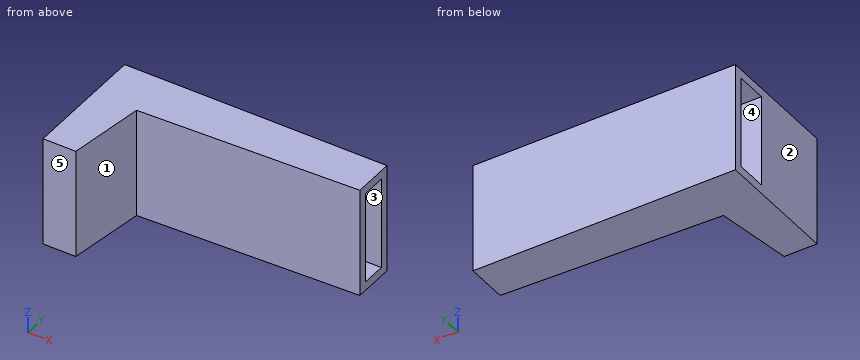
from build123d import *

# Parameters (mm, degrees)
PAD001_DEPTH = 8.4
PAD_DEPTH    = 10


with BuildPart() as pegcutoutpad:
    # Sketch001 → Pad001 (new body)
    with BuildSketch(Plane.XY.offset(0.8)):
        Polygon((20, -0.8), (-4, -0.8), (-4, -3.67), (0, -3.67), (20, -3.016154), align=None)
    extrude(amount=PAD001_DEPTH)


with BuildPart() as pegcut:
    # Sketch → Pad (new body)
    with BuildSketch(Plane.XY):
        Polygon((20, 0), (20, -3.816154), (0, -4.47), (-1, -11.47), (-4, -11.47), (-4, 0), align=None)
    extrude(amount=PAD_DEPTH)

    # Cut: cut PegCutOutPad
    add(pegcutoutpad.part, mode=Mode.SUBTRACT)


solid = pegcut.part
Part model, mm, in its own coordinate system. Face numbers are marked on the shaded views. A direction names the side the tool comes from. Give positions to 0.01 mm unless a question says otherwise; leave off trailing zeros. Order: outer loops, then holes, each group sorted by start corner. A loop starts at its lowest first (then second) coordinate and runs counter-clockwise, first axis right, second up. Notation, with made-up numbers: (-23, 41) -> (-8, 41) arc R16 cw to (-8, 50) -> close; hole circle Ø8 at (-40, 21). An arc over 180 degrees is marked (long way). Use one line per item in the form item = value.
(1) Pull direction Y, two halves, no side cores. Call the marked faces 1, 2 and 3: +Y half, -Y half, draft (parallel to the pull), parting line (faces both ways), or undercut.
Solution:
face_1 = -Y half
face_2 = draft
face_3 = undercut
(2) Tool access for the marked faces 4 and 5: list every direction of +Z, -Z, +X, -X, +Y, -Y with a clear straight run to the whole face (end or side of a thin tool).
Solution:
face_4 = -X
face_5 = +Z, -Z, +X, -X, -Y
(3) Drill centre lines: line 1 (Z direction, x = 13.25, y = -2); line 2 (Y direction, x = 18.25, z = 3); line 3 (Y direction, x = 11.75, z = 9). Where is each one in solid material? Low to high. Write a range as from..to.
Solution:
line_1 = 0..0.8, 9.2..10
line_2 = -3.87..-3.07, -0.8..0
line_3 = -4.09..-3.29, -0.8..0
(4) Saw through at B-B (x = -2). Write the cut outline in (y, z), then the cut area to 3 significant figures.
Solution:
outline = (-11.47, 0) -> (0, 0) -> (0, 10) -> (-11.47, 10) -> close; hole (-3.67, 0.8) -> (-0.8, 0.8) -> (-0.8, 9.2) -> (-3.67, 9.2) -> close
area = 90.6 mm²
(5) Saw through at C-C (x = 12.75). Write the cut outline in (y, z), then the cut area to 3 significant figures.
Solution:
outline = (-4.05, 0) -> (0, 0) -> (0, 10) -> (-4.05, 10) -> close; hole (-3.25, 0.8) -> (-0.8, 0.8) -> (-0.8, 9.2) -> (-3.25, 9.2) -> close
area = 19.9 mm²
(6) Saw through at A-A (z = 3). Write the cut outline in (x, y), then the cut area to 3 significant figures.
Solution:
outline = (-4, -11.47) -> (-1, -11.47) -> (0, -4.47) -> (20, -3.82) -> (20, -3.02) -> (0, -3.67) -> (-4, -3.67) -> close; (-4, -0.8) -> (20, -0.8) -> (20, 0) -> (-4, 0) -> close
area = 62.9 mm²
(7) Saw through at D-D (y = -5.25). Write the cut outline in (x, z).
Solution:
outline = (-4, 0) -> (-0.11, 0) -> (-0.11, 10) -> (-4, 10) -> close
(8) Flat gauge pins, fed straight in: P1, Ø2, axis at x = 0, y = -5, coming from the +Z side; P2, Ø6, axis at x = 14, z = 5, coming from the -Y side; P3, Ø4, axis at y = -9.5, z = 4, coming from the +X side; P4, Ø4, axis at x = 16, z = 3, coming from the -Y side. Where does each tip first touch, or does it go through?
Solution:
P1 = 10
P2 = -4.11
P3 = -0.43
P4 = -4.01
